```python
from build123d import *

# Parameters (mm, degrees)
BALAYAGE_MINCE1_PROFILE_R   = 3
BALAYAGE_MINCE1_PROFILE_R_2 = 2


with BuildPart() as part:
    # Balayage-Mince1: sweep along a curve in space
    with BuildLine() as balayage_mince1_path:
        Line((14, 165, -59.25), (14, 207.375, -59.25))
        ThreePointArc((14, 207.375, -59.25), (45.407462351, 238.890799577, -56.639074556), (76.814924701, 207.375, -54.028149113))
        Line((76.814924701, 207.375, -54.028149113), (76.814924701, 81.65, -54.028149113))
    # Balayage-Mince1 profile (on start of the path) → Balayage-Mince1 (sweep)
    with BuildSketch(Plane(origin=(14, 165, -59.25), x_dir=(0, 0, 1), z_dir=(0, 1, 0))):
        Circle(BALAYAGE_MINCE1_PROFILE_R)
        Circle(BALAYAGE_MINCE1_PROFILE_R_2, mode=Mode.SUBTRACT)
    sweep(path=balayage_mince1_path.line)


solid = part.part
```
Part model, mm, in its own coordinate system. A direction names the side the tool comes from. Give positions to 0.01 mm unless a question says otherwise; leave off trailing zeros. Write each loop counter-clockwise with the first axis right and the second up, starting at its lowest first coordinate (ties: lowest second). Pieces come first, ordered by that corner, then holes. Notation, with made-up numbers: (72.25, 15) -> (103.25, 15) arc R9 ccw to (103.25, 21) -> close; hole circle Ø1 at (-20.5, -34.75). An arc over 180 degrees is marked (long way). Put each result on its own line as item: value. Start each with the question number.
Item 1: Wall check: L1, parallel to Z at x = 76.5, y = 187.5; L2, parallel to X at y = 103, z = -55.5; L3, parallel to X at y = 140, z = -53.5. Give the ranges that are in metal, low to high. Write a range as [from, to].
Item 2: Pull direction X, two halves, no side cores. Call faces 3 (the face through (13, 165, -57)), 4 (the face through (78.41, 143.63, -52.82)): pulls with the +X half, pulls with the -X half, needs draft (parallel to the pull), parting line crosses it, or undercut.
Item 3: Cut at A-A (y = 181.5). List the corners of the cut face in (x, z), then the cut area to 3 significant figures.
Item 4: Pin check, flat tips, straight feed: pin 1 Ø3 at (x, z) = (12.5, -58.5) entering from -Y; pin 2 Ø6 at (y, z) = (140.5, -57) entering from -X; pin 3 Ø3 at (x, z) = (14, -59.25) entering from +Y. Stop position of each tip, or through.
Item 5: Which spindle directions (+Z, -Z, +X, -X, +Y, -Y) get a long thin tool onto all of the face, cutting with end or side? Do faces 1 (the face through (78, 81.65, -56)), 2 (the face through (14.601, 186.484, -57.342)). Say none if no direction does.
Item 6: Cut at B-B (y = 110.5). List the corners of the cut face in (x, z).
Answer list:
1. L1: z = [-57.01, -56], [-52.05, -51.04]
1. L2: x = [74.2, 75.46], [78.17, 79.43]
1. L3: x = [73.86, 74.89], [78.74, 79.77]
2. face 3: needs draft
2. face 4: undercut
3. outline: circle Ø6 at (14, -59.25); circle Ø6 at (76.81, -54.03); hole circle Ø4 at (14, -59.25); hole circle Ø4 at (76.81, -54.03)
3. area: 31.4 mm2
4. pin 1: stops at y = 165
4. pin 2: stops at x = 73.81
4. pin 3: stops at y = 224.42
5. face 1: +Z, -Z, +X, -X, -Y
5. face 2: -Y
6. outline: circle Ø6 at (76.81, -54.03); hole circle Ø4 at (76.81, -54.03)
